```python
from build123d import *

# Parameters (mm, degrees)
SKETCH1_R           = 5
BOSS_EXTRUDE1_DEPTH = 80
CHAMFER1_SIZE       = 5
FILLET1_R           = 1


with BuildPart() as part:
    # Sketch1 → Boss-Extrude1 (new body)
    with BuildSketch(Plane(origin=(0, 0, 0), x_dir=(1, 0, 0), z_dir=(0, 1, 0))):
        with Locations(Location((0, 0, 0), (0, 0, 270))):
            Circle(SKETCH1_R)
    extrude(amount=BOSS_EXTRUDE1_DEPTH)

    # Chamfer1
    chamfer1_edges = [part.edges().sort_by_distance(p)[0] for p in [
        (0, 0, -5),
    ]]
    chamfer(chamfer1_edges, length=CHAMFER1_SIZE)

    # Fillet1
    fillet1_edges = [part.edges().sort_by_distance(p)[0] for p in [
        (0, 80, -5),
    ]]
    fillet(fillet1_edges, radius=FILLET1_R)


solid = part.part
```
Geometry check sheet. Reference: the model listing, model coordinates, mm. Give positions to 0.01 mm unless a question says otherwise; leave off trailing zeros. Loops run counter-clockwise (first coordinate to the right, second up) from the corner with the lowest first, then second, coordinate; pieces in that order, holes last. Notation, with made-up numbers: M -12,87.5 L 6,87.5 A31 cw 6,123.5 Z; hole C 3,18.25 d7. An arc over 180 degrees is marked long. Write item = value, one per line.
(1) Material ranges on line 1 (Z direction, x = -0.25, y = 74.5); line 2 (Z direction, x = 3, y = 29); line 3 (Y direction, x = -2.25, z = 3), recorded low to high. Write a range as [from, to].
Answer below:
line_1 = [-4.99, 4.99]
line_2 = [-4, 4]
line_3 = [3.75, 80]
(2) Gauge pin test, flat ends, axial feed: pin 1 Ø1.5 at (x, y) = (-3.5, 41.5) entering from +Z; pin 2 Ø1.5 at (x, y) = (2, 45.5) entering from -Z; pin 3 Ø4 at (x, y) = (-3, 55.5) entering from -Z. Record the tip position at first contact, or that the pin passes through.
Answer below:
pin_1 = 4.18
pin_2 = -4.84
pin_3 = -4.9
(3) Sectioned sample at A-A, the plane y = 74. Record the cut outline in (x, z), plus the area to 3 significant figures.
Answer below:
outline = C 0,0 d10
area = 78.5 mm2
